Read the model definition and answer for the solid it produces. Units are mm, in the model's axes. Face numbers are marked on the shaded views. Give positions to 0.01 mm unless a question says otherwise; leave off trailing zeros. Order: outer loops, then holes, each group sorted by start corner. A loop starts at its lowest first (then second) coordinate and runs counter-clockwise, first axis right, second up. Notation, with made-up numbers: (-30, -13) - (-5, -13) arc R13 ccw to (-5, -9) - close; hole circle Ø5 at (-11.5, -34.75). An arc over 180 degrees is marked (long way). Return JSON: item names as keys, results as strings.
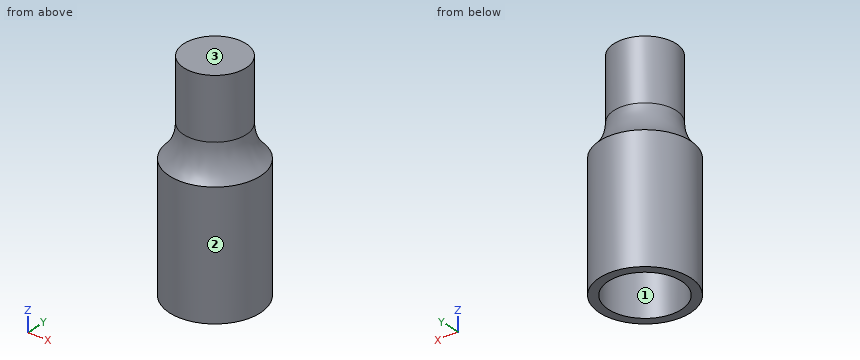
```python
from build123d import *


# Not quite as in the source:
# - a fillet or chamfer that OpenCascade refuses, or shapes differently, is made with other operations: its cross-section is extruded or revolved along the edge and cut away or added


with BuildPart() as f1:
    # F0 (on Front) → F1 (revolve)
    with BuildSketch(Plane.XZ):
        Polygon((4.1, -14), (5.1, -14), (5.1, 0), (3.5, 0), (3.5, 10.5), (0, 10.5), (0, 10), (2.7, 10), (2.7, -2), (4.1, -2), align=None)
    revolve(axis=Axis((0, 0, -6.7832856439), (0, 0, -1)))

    # F2: fillet of radius 5 on 1 edges, made by hand

    # F2_s1 → F2_t2 (revolve)
    with BuildSketch(Plane.XZ):
        with BuildLine():
            ThreePointArc((5.1, 0), (3.917424305, 1.666060556), (3.5, 3.666060556))
            Line((3.5, 3.666060556), (3.5, 0))
            Line((3.5, 0), (5.1, 0))
        make_face()
    revolve(axis=Axis((0, 0, 0), (0, 0, -1)))


solid = f1.part
```
Q1. Consider L1, parallel to X at y = 0, z = -7.75; L2, parallel to Z at x = -2.5, y = -0.75. Determine where each line is inside the solid, lowest interval first.
Values:
{"L1": "x = -5.1 to -4.1, 4.1 to 5.1", "L2": "z = 10 to 10.5"}
Q2. A cutting plane is placed at B-B (z = 4.5). Write down the section's boundary in (x, y).
Values:
{"outline": "circle Ø7 at (0, 0); hole circle Ø5.4 at (0, 0)"}
Q3. Given pin 1 (1.5 mm diameter, centred on x = -4, z = -7, fed in from +Y); pin 2 (2.5 mm diameter, centred on x = -1.5, y = 0.5, fed in from -Z); pin 3 (3 mm diameter, centred on x = -3.5, z = -9, fed in from -Y), each flat-ended and moving along its own axis, determine where each tip first touches the part or whether it passes through.
Values:
{"pin 1": "stops at y = 3.93", "pin 2": "stops at z = -2", "pin 3": "stops at y = -4.69"}
Q4. A cutting plane is placed at D-D (z = -10.5). Write down the section's boundary in (x, y), and give its area (3 significant figures).
Values:
{"outline": "circle Ø10.2 at (0, 0); hole circle Ø8.2 at (0, 0)", "area": "28.9 mm²"}
Q5. A cutting plane is placed at A-A (x = 0). Write down the section's boundary in (y, z).
Values:
{"outline": "(-5.1, -14) - (-4.1, -14) - (-4.1, -2) - (-2.7, -2) - (-2.7, 10) - (2.7, 10) - (2.7, -2) - (4.1, -2) - (4.1, -14) - (5.1, -14) - (5.1, 0) arc R5 cw to (3.5, 3.67) - (3.5, 10.5) - (-3.5, 10.5) - (-3.5, 3.67) arc R5 cw to (-5.1, 0) - close"}
Q6. Determine the mould class of the marked faces 1, 2 and 3 for opening direction X: released by +X, released by -X, zero draft, split by the parting line, or undercut.
Values:
{"face 1": "undercut", "face 2": "split by the parting line", "face 3": "zero draft"}
